Here's how the part is built. I have some questions about the finished solid (model axes, mm). Face numbers are marked on the shaded views. A direction names the side the tool comes from. Give positions to 0.01 mm unless a question says otherwise; leave off trailing zeros. Order: outer loops, then holes, each group sorted by start corner. A loop starts at its lowest first (then second) coordinate and runs counter-clockwise, first axis right, second up. Notation, with made-up numbers: M 35,-22 L 46,-22 A19 ccw 46,0 Z; hole C -7.75,28 d6. An arc over 180 degrees is marked long. One line per item, written item: value. Start each with the question number.
from build123d import *

# Parameters (mm, degrees)
BOSS_EXTRU_2_DEPTH      = 5
ESQUISSE3_R             = 1.75
ENL_V_MAT_EXTRU_2_DEPTH = 4
ESQUISSE4_R             = 3.5
ENL_V_MAT_EXTRU_3_DEPTH = 12.5


with BuildPart() as part:
    # Esquisse1 → Boss.-Extru.2 (new body)
    with BuildSketch(Plane.XY):
        with BuildLine():
            Line((-20, 0.5), (-14.585952146, 0.5))
            ThreePointArc((-14.585952146, 0.5), (-12.728534584, 1.144156202), (-11.668761717, 2.8))
            ThreePointArc((-11.668761717, 2.8), (0, 12), (11.668761717, 2.8))
            ThreePointArc((11.668761717, 2.8), (12.728534584, 1.144156202), (14.585952146, 0.5))
            Line((14.585952146, 0.5), (20, 0.5))
            Line((20, 0.5), (20, 3.5))
            Line((20, 3.5), (14.585952146, 3.5))
            ThreePointArc((14.585952146, 3.5), (0, 15), (-14.585952146, 3.5))
            Line((-14.585952146, 3.5), (-20, 3.5))
            Line((-20, 3.5), (-20, 0.5))
        make_face()
    extrude(amount=BOSS_EXTRU_2_DEPTH)

    # Esquisse3 → Enlèv. mat.-Extru.2 (cut, through all)
    with BuildSketch(Plane(origin=(0, 3.5, 0), x_dir=(1, 0, 0), z_dir=(0, 1, 0))):
        with Locations((-17, -2.5)):
            Circle(ESQUISSE3_R)
        with Locations((17, -2.5)):
            Circle(ESQUISSE3_R)
    extrude(amount=-ENL_V_MAT_EXTRU_2_DEPTH, mode=Mode.SUBTRACT)

    # Esquisse4 → Enlèv. mat.-Extru.3 (cut, through all)
    with BuildSketch(Plane(origin=(0, 3.5, 0), x_dir=(1, 0, 0), z_dir=(0, 1, 0))):
        with Locations((-17, -2.5)):
            Circle(ESQUISSE4_R)
        with Locations((17, -2.5)):
            Circle(ESQUISSE4_R)
    extrude(amount=ENL_V_MAT_EXTRU_3_DEPTH, mode=Mode.SUBTRACT)


solid = part.part
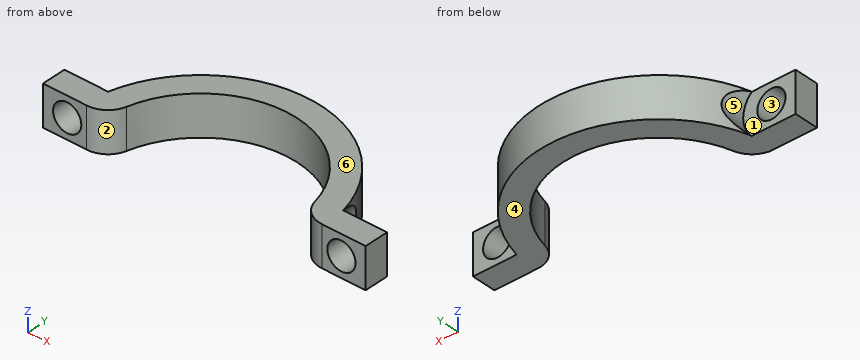
Item 1: I want a section at B-B on x = 17. Write out the boundary of the cut face in (y, z).
Item 2: Will these pins go through, and if not, where does the flat tip stop? P1, Ø1, axis at y = 4.5, z = 3, coming from the -X side; P2, Ø2, axis at y = 9.5, z = 3.5, coming from the +X side; P3, Ø3, axis at y = 5.5, z = 3, coming from the -X side; P4, Ø3, axis at x = 17, z = 2.5, coming from the -Y side.
Item 3: Please list where these lines run through material, in increasing order: probe 1 along Z at (x, y) = (-17, 1.95); probe 2 along X at (y, z) = (3.25, 1.8); probe 3 along X at (y, z) = (1.65, 2.5). Write a range as [from, to].
Item 4: I want a section at D-D on x = 0.5. Write out the boundary of the cut face in (y, z).
Item 5: I want a section at A-A on z = 2.5. Write out the boundary of the cut face in (x, y).
Item 6: We'd pull the mould along Z, two halves only. Please class the marked faces 4, 5 and 6: +Z half, -Z half, draft (parallel to the pull), parting line (faces both ways), or undercut.
Item 7: I want a section at C-C on y = 13.75. Write out the boundary of the cut face in (x, z).
Item 8: For the marked faces 1, 2 and 3, which set-ups out of +Z, -Z, +X, -X, +Y, -Y let a thin tool reach every point of the face, with its end or its side?
Answer below:
1. outline: M 0.5,0 L 3.5,0 L 3.5,0.75 L 0.5,0.75 Z; M 0.5,4.25 L 3.5,4.25 L 3.5,5 L 0.5,5 Z
2. P1: stops at x = -13.65
2. P2: stops at x = 12.36
2. P3: stops at x = -14.1
2. P4: passes through
3. probe 1: z = [0, 0.75], [4.25, 5]
3. probe 2: x = [-20, -18.6], [-15.4, -11.55], [11.55, 15.4], [18.6, 20]
3. probe 3: x = [-20, -18.75], [-15.25, -12.22], [12.22, 15.25], [18.75, 20]
4. outline: M 11.99,0 L 14.99,0 L 14.99,5 L 11.99,5 Z
5. outline: M -20,0.5 L -18.75,0.5 L -18.75,3.5 L -20,3.5 Z; M -15.25,0.5 L -14.59,0.5 A3 ccw -11.67,2.8 A12 cw 11.67,2.8 A3 ccw 14.59,0.5 L 15.25,0.5 L 15.25,3.5 L 13.5,3.5 L 13.5,6.54 A15 ccw -13.5,6.54 L -13.5,3.5 L -15.25,3.5 Z; M 18.75,0.5 L 20,0.5 L 20,3.5 L 18.75,3.5 Z
6. face 4: -Z half
6. face 5: undercut
6. face 6: +Z half
7. outline: M -5.99,0 L 5.99,0 L 5.99,5 L -5.99,5 Z
8. face 1: -X, +Y
8. face 2: +Z, -Z, -Y
8. face 3: +Y, -Y
